Build history of the part. All positions in model axes, mm. A direction names the side the tool comes from. Give positions to 0.01 mm unless a question says otherwise; leave off trailing zeros. Order: outer loops, then holes, each group sorted by start corner. A loop starts at its lowest first (then second) coordinate and runs counter-clockwise, first axis right, second up. Notation, with made-up numbers: (82.25, -16) - (113.25, -16) arc R13 cw to (113.25, -4) - close; hole circle Ø9 at (55.5, -17.75). An arc over 180 degrees is marked (long way). Write each question's results on one line, items separated by ' | '. Start each with the question number.
1) Drop flat-ended pins along their axis: pin 1 Ø0.6 at (y, z) = (164.5, 70) entering from -X; pin 2 Ø1.6 at (x, y) = (-28, 163) entering from +Z; pin 3 Ø3 at (y, z) = (159.5, 19.5) entering from +X. Give the stop position or say it passes through.
2) Drill centre lines: line 1 along Y through (x, z) = (3, -2.5); line 2 along Z through (x, y) = (7, 158.5). Where is each one in solid material? Low to high. Write a range as from..to.
3) Cut at B-B on x = -20. List the corners of the cut face in (y, z).
4) Tool access for faces 5 (the face through (38, 78, -1)), 6 (the face through (1, 78, 90)), 7 (the face through (-37, 159, -1)), 8 (the face through (-1, 159, 89)), 9 (the face through (37, 159, 1)): list every direction of +Z, -Z, +X, -X, +Y, -Y with a clear straight run to the whole face (end or side of a thin tool).
5) Cut at D-D on x = -29. List the corners of the cut face in (y, z).
6) Two-plate mould, pull along Y, no slides. Class faces 1 (the face through (-29, 164, 72)), 2 (the face through (1, 0, 1)), 3 (the face through (1, 159, -89)), 4 (the face through (-29, 165, 72)): +Y half, -Y half, draft (parallel to the pull), parting line (faces both ways), or undercut.
7) Cut at C-C on z = -5. List the corners of the cut face in (x, y), plus the area to 3 significant figures.
8) Cut at A-A on z = 70. List the corners of the cut face in (x, y).
Autodesk Inventor part; units mm, degrees
ref_plane "YZ Plane" through (0, 0, 0) normal (1, 0, 0) x (0, 1, 0)
ref_plane "XZ Plane" through (0, 0, 0) normal (0, 1, 0) x (-1, 0, 0)
ref_plane "XY Plane" through (0, 0, 0) normal (0, 0, 1) x (1, 0, 0)
sketch "Sketch1" plane through (0, 0, 0) normal (0, 1, 0) x (-1, 0, 0)
  line L0 (-38, 90) -> (38, 90)
  line L1 (38, 90) -> (38, -90)
  line L2 (38, -90) -> (-38, -90)
  line L3 (-38, -90) -> (-38, 90)
  line L4 (-38, 90) -> (38, -90) construction
  line L5 (38, 90) -> (-38, -90) construction
  point P0 (0, 0)
  dimension "d0" = 76
  dimension "d1" = 180
extrude "Extrusion1" add sketch "Sketch1" along normal blind 162
sketch "Sketch2" plane through (0, 162, 0) normal (0, 1, 0) x (1, 0, 0)
  line L0 (-38, -90) -> (38, -90) construction
  line L1 (38, -90) -> (38, 90) construction
  line L2 (38, 90) -> (-38, 90) construction
  line L3 (-38, 90) -> (-38, -90) construction
  line L4 (-37, -89) -> (37, -89)
  line L5 (37, -89) -> (37, 89)
  line L6 (37, 89) -> (-37, 89)
  line L7 (-37, 89) -> (-37, -89)
  line L8 (-38, 90) -> (-38, -90)
  line L9 (-38, -90) -> (38, -90)
  line L10 (38, -90) -> (38, 90)
  line L11 (38, 90) -> (-38, 90)
  line L12 (-38, 90) -> (-38, -90)
  point P0 (0, 0)
  dimension "d4" = 1
extrude "Extrusion2" cut sketch "Sketch2" against normal blind 5
fillet "Fillet1" radius 1 16 edges at (38, 78.5, -90) (38, 78.5, 90) (-38, 78.5, -90) (-38, 78.5, 90) (0, 0, 90) (-38, 0, 0) (0, 0, -90) (38, 0, 0) (37, 159.5, -89) (37, 162, 0) (0, 162, -89) (37, 159.5, 89) (-37, 159.5, 89) (0, 162, 89) (-37, 162, 0) (-37, 159.5, -89)
sketch "Sketch3" plane through (0, 162, 0) normal (0, 1, 0) x (1, 0, 0)
  line L0 (37, -88) -> (37, 88) construction
  line L1 (-36, -89) -> (36, -89) construction
  line L2 (-37, 88) -> (-37, -88) construction
  line L3 (-32, -78) -> (-26, -78)
  line L4 (-26, -78) -> (-26, -77)
  line L5 (-26, -77) -> (-32, -77)
  line L6 (-32, -77) -> (-32, -78)
  line L7 (-32, -78) -> (-26, -77) construction
  line L8 (-26, -78) -> (-32, -77) construction
  line L9 (26, -78) -> (32, -78)
  line L10 (32, -78) -> (32, -77)
  line L11 (32, -77) -> (26, -77)
  line L12 (26, -77) -> (26, -78)
  line L13 (26, -78) -> (32, -77) construction
  line L14 (32, -78) -> (26, -77) construction
  point P0 (0, 0)
  point P1 (-29, -77.5)
  point P2 (29, -77.5)
  dimension "d12" = 6
  dimension "d13" = 1
  dimension "d14" = 6
  dimension "d15" = 1
  dimension "d16" = 11
  dimension "d17" = 5
  dimension "d18" = 5
  dimension "d19" = 11
extrude "Extrusion3" add sketch "Sketch3" along normal blind 3
sketch "Sketch4" plane through (32, 162, 77) normal (0, 0, -1) x (-1, 0, 0)
  line L0 (-0.25, 2) -> (6.25, 2)
  line L1 (6.25, 2) -> (6.25, 3)
  line L2 (6.25, 3) -> (-0.25, 3)
  line L3 (-0.25, 3) -> (-0.25, 2)
  line L4 (-0.25, 2) -> (6.25, 3) construction
  line L5 (6.25, 2) -> (-0.25, 3) construction
  line L6 (0, 3) -> (6, 3) construction
  line L7 (57.75, 2) -> (64.25, 2)
  line L8 (64.25, 2) -> (64.25, 3)
  line L9 (64.25, 3) -> (57.75, 3)
  line L10 (57.75, 3) -> (57.75, 2)
  line L11 (57.75, 2) -> (64.25, 3) construction
  line L12 (64.25, 2) -> (57.75, 3) construction
  line L13 (58, 3) -> (64, 3) construction
  point P0 (32, -162)
  point P1 (3, 2.5)
  point P2 (3, 3)
  point P3 (61, 2.5)
  point P4 (61, 3)
  dimension "d22" = 6.5
  dimension "d23" = 1
  dimension "d24" = 6.5
  dimension "d25" = 1
extrude "Extrusion4" add sketch "Sketch4" along normal blind 10
fillet "Fillet2" radius 0.25 28 edges at (32.25, 164.5, 67) (25.75, 164.5, 67) (32.25, 164.5, 77) (25.75, 164.5, 77) (-25.75, 164.5, 67) (-25.75, 164.5, 77) (-32.25, 164.5, 67) (-32.25, 164.5, 77) (-32.25, 165, 72) (-32.25, 164, 72) (-29, 165, 67) (-29, 164, 67) (-25.75, 164, 72) (-25.75, 165, 72) (-26, 163, 77) (-26, 163.5, 78) (-32, 163, 77) (-32, 163.5, 78) (32.25, 165, 72) (32.25, 164, 72) (32, 163, 77) (32, 163.5, 78) (29, 165, 67) (29, 164, 67) (25.75, 165, 72) (25.75, 164, 72) (26, 163, 77) (26, 163.5, 78)
fillet "Fillet2" radius 1 2 edges at (29, 165, 78) (-29, 165, 78)
properties part number "NP18-12 Battery" material "Copper"
Results:
1) pin 1: x = -32.25 | pin 2: z = 78 | pin 3: x = 37
2) line 1: 0..162 | line 2: -89..89
3) outline: (0, -89) arc R1 ccw to (1, -90) - (157, -90) - (157, -89) - (161, -89) arc R1 ccw to (162, -88) - (162, 88) arc R1 ccw to (161, 89) - (157, 89) - (157, 90) - (1, 90) arc R1 ccw to (0, 89) - close
4) face 5: +Z, -Z, +X, +Y, -Y | face 6: +Z, +X, -X, +Y, -Y | face 7: +Z, -Z, -X, +Y | face 8: +Z, +X, -X, +Y | face 9: +Z, -Z, +X, +Y
5) outline: (0, -89) arc R1 ccw to (1, -90) - (157, -90) - (157, -89) - (161, -89) arc R1 ccw to (162, -88) - (162, 77) - (164, 77) - (164, 67.25) arc R0.25 ccw to (164.25, 67) - (164.75, 67) arc R0.25 ccw to (165, 67.25) - (165, 77) arc R1 ccw to (164, 78) - (162, 78) - (162, 88) arc R1 ccw to (161, 89) - (157, 89) - (157, 90) - (1, 90) arc R1 ccw to (0, 89) - close
6) face 1: undercut | face 2: -Y half | face 3: draft | face 4: +Y half
7) outline: (-38, 1) arc R1 ccw to (-37, 0) - (37, 0) arc R1 ccw to (38, 1) - (38, 157) - (37, 157) - (37, 161) arc R1 ccw to (36, 162) - (-36, 162) arc R1 ccw to (-37, 161) - (-37, 157) - (-38, 157) - close | area: 12,300 mm^2
8) outline: (-38, 1) arc R1 ccw to (-37, 0) - (37, 0) arc R1 ccw to (38, 1) - (38, 157) - (37, 157) - (37, 161) arc R1 ccw to (36, 162) - (-36, 162) arc R1 ccw to (-37, 161) - (-37, 157) - (-38, 157) - close; (-32.25, 164.25) arc R0.25 ccw to (-32, 164) - (-26, 164) arc R0.25 ccw to (-25.75, 164.25) - (-25.75, 164.75) arc R0.25 ccw to (-26, 165) - (-32, 165) arc R0.25 ccw to (-32.25, 164.75) - close; (25.75, 164.25) arc R0.25 ccw to (26, 164) - (32, 164) arc R0.25 ccw to (32.25, 164.25) - (32.25, 164.75) arc R0.25 ccw to (32, 165) - (26, 165) arc R0.25 ccw to (25.75, 164.75) - close
